Can you work these out from the model? Positions are in its coordinate system, mm. Face numbers are marked on the shaded views. A direction names the side the tool comes from. Round coordinates to 2 decimals unless told otherwise and drop trailing zeros. Write each loop counter-clockwise with the first axis right and the second up, starting at its lowest first coordinate (ties: lowest second). Pieces come first, ordered by that corner, then holes. Notation, with made-up numbers: M -12,14 L 14,14 A24 ccw 14,44 Z; hole C 83.25,-7.75 d3. An arc over 180 degrees is marked long. Answer in a Markdown table with one row per item. Add a question column.
(1) If I drill on probe 1 along X at (y, z) = (-0.5, -5.5); probe 2 along Y at (x, z) = (0.25, 0); probe 3 along X at (y, z) = (0.75, -4.75), over which ranges is the centre line in solid material (lowest first)?
(2) I'm going to push flat-ended pins straight in: pin 1 (1 mm diameter, centred on x = 0.5, y = -1, fed in from +Z); pin 2 (3 mm diameter, centred on x = -1, z = -4, fed in from -Y); pin 3 (2 mm diameter, centred on x = -1, z = -3, fed in from -Y). Where does each tip first touch, or does it pass through?
(3) For the marked faces 1, 2 and 3, which set-ups out of +Z, -Z, +X, -X, +Y, -Y let a thin tool reach every point of the face, with its end or its side?
(4) Suppose I cut it at C-C, the plane x = 0.2. Write out the boundary of the cut face in (y, z), then the cut area to 3 significant figures.
(5) If we mould it in two halves opening along X, with no side actions, what happens to the marked faces 4, 5 and 6? For each: released by +X, released by -X, zero draft, split by the parting line, or undercut.
(6) Suppose I cut it at D-D, the plane x = -1.65. Write out the boundary of the cut face in (y, z) (1 decimal), then the cut area to 3 significant figures.
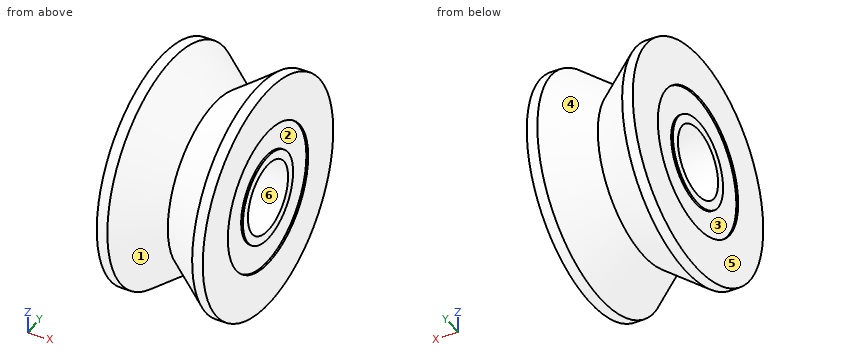
from build123d import *

# Parameters (mm, degrees)
SKETCH2_R          = 4
SKETCH2_R_2        = 2.5
CUT_EXTRUDE1_DEPTH = 0.1


with BuildPart() as part:
    # Sketch1 → Revolve1 (revolve)
    with BuildSketch(Plane.XY, mode=Mode.PRIVATE) as revolve1_sk:
        Polygon((-3, 2), (3, 2), (3, 6.5), (2.4, 6.5), (0, 4.7), (-2.4, 6.5), (-3, 6.5), align=None)
    revolve(revolve1_sk.sketch.rotate(Axis((0, 0, 0), (1, 0, 0)), 90), axis=Axis((0, 0, 0), (1, 0, 0)))

    # Sketch2 → Cut-Extrude1 (cut)
    with BuildSketch(Plane(origin=(3, 0, 0), x_dir=(0, 0, -1), z_dir=(1, 0, 0))):
        Circle(SKETCH2_R)
        Circle(SKETCH2_R_2, mode=Mode.SUBTRACT)
    cut_extrude1 = extrude(amount=-CUT_EXTRUDE1_DEPTH, mode=Mode.SUBTRACT)

    # Mirror1: Cut-Extrude1 across plane
    add(cut_extrude1.mirror(Plane(origin=(0, 0, 0), x_dir=(0, 0, 1), z_dir=(1, 0, 0))), mode=Mode.SUBTRACT)


solid = part.part
Calculated:
| question | item | result |
|---|---|---|
| 1 | probe 1 | -3 to -1.1, 1.1 to 3 |
| 1 | probe 2 | -4.89 to -2, 2 to 4.89 |
| 1 | probe 3 | -3 to -0.15, 0.15 to 3 |
| 2 | pin 1 | z = 5.37 |
| 2 | pin 2 | y = -5.54 |
| 2 | pin 3 | y = -5.56 |
| 3 | face 1 | none |
| 3 | face 2 | +X |
| 3 | face 3 | -X |
| 4 | outline | C 0,0 d9.7; hole C 0,0 d4 |
| 4 | area | 61.3 mm² |
| 5 | face 4 | undercut |
| 5 | face 5 | released by -X |
| 5 | face 6 | zero draft |
| 6 | outline | C 0,0 d11.9; hole C 0,0 d4 |
| 6 | area | 98.2 mm² |
